```python
from build123d import *

# Parameters (mm, degrees)
F0_W     = 700
F0_H     = 800
F0_W_2   = 10
F0_H_2   = 301
F1_DEPTH = 5
F2_W     = 94.870865
F2_H     = 35.080195
F3_DEPTH = 25


with BuildPart() as f1:
    # F0 (on Top) → F1 (new body)
    with BuildSketch(Plane.XY):
        Rectangle(F0_W, F0_H)
        with Locations((-103, 5.5)):
            Rectangle(F0_W_2, F0_H_2, mode=Mode.SUBTRACT)
    extrude(amount=F1_DEPTH)

    # F2 (on face) → F3 (join)
    with BuildSketch(Plane.XY):
        with Locations((180.280223, -316.02779)):
            Rectangle(F2_W, F2_H)
    extrude(amount=-F3_DEPTH)


solid = f1.part
```
Check sheet for the modelled part. Datum: model origin and axes. Units: mm. A direction names the side the tool comes from. Give positions to 0.01 mm unless a question says otherwise; leave off trailing zeros. Loops run counter-clockwise (first coordinate to the right, second up) from the corner with the lowest first, then second, coordinate; pieces in that order, holes last. Notation, with made-up numbers: M -9.5,-6.5 L 45.5,-6.5 A15 ccw 45.5,4.5 Z; hole C 15.5,-20 d3. An arc over 180 degrees is marked long. Answer as CSV lines item,"result".
Item 1: Set-up check for faces 1 (the face through (180, -298.488, -12)), 2 (the face through (180, -333.568, -12)), 3 (the face through (132.845, -316, -12)): record each of +Z, -Z, +X, -X, +Y, -Y from which the full face is reachable in a straight line by a thin tool's end or side.
Reply:
face 1,"-Z, +X, -X, +Y"
face 2,"-Z, +X, -X, -Y"
face 3,"-Z, -X, +Y, -Y"
Item 2: Sectioned sample at B-B, the plane z = -8.25. Enter the section's corners in (x, y), then the cut area to 3 significant figures.
Reply:
outline,"M 132.84,-333.57 L 227.72,-333.57 L 227.72,-298.49 L 132.84,-298.49 Z"
area,"3,330 mm^2"
Item 3: Scan lines: L1, parallel to Z at x = -44.5, y = -96; L2, parallel to Y at x = 206.5, z = -20; L3, parallel to X at y = -328.5, z = -3.5. Record each from-to range of solid material in increasing order.
Reply:
L1,"0 to 5"
L2,"-333.57 to -298.49"
L3,"132.84 to 227.72"
Item 4: Sectioned sample at A-A, the plane y = 104. Enter the section's corners in (x, z).
Reply:
outline,"M -350,0 L -108,0 L -108,5 L -350,5 Z; M -98,0 L 350,0 L 350,5 L -98,5 Z"
Item 5: Sectioned sample at C-C, the plane x = 89. Enter the section's corners in (y, z), then the cut area to 3 significant figures.
Reply:
outline,"M -400,0 L 400,0 L 400,5 L -400,5 Z"
area,"4,000 mm^2"
Item 6: Depth check by flat-ended pin: pin 1 Ø6 at (x, y) = (-91.5, 134) entering from -Z; pin 2 Ø12.5 at (y, z) = (-320.5, -13.5) entering from +X; pin 3 Ø7.5 at (y, z) = (-308.5, -16) entering from -X. Enter the tip coordinate at first touch or a pass-through.
Reply:
pin 1,"z = 0"
pin 2,"x = 227.72"
pin 3,"x = 132.84"
